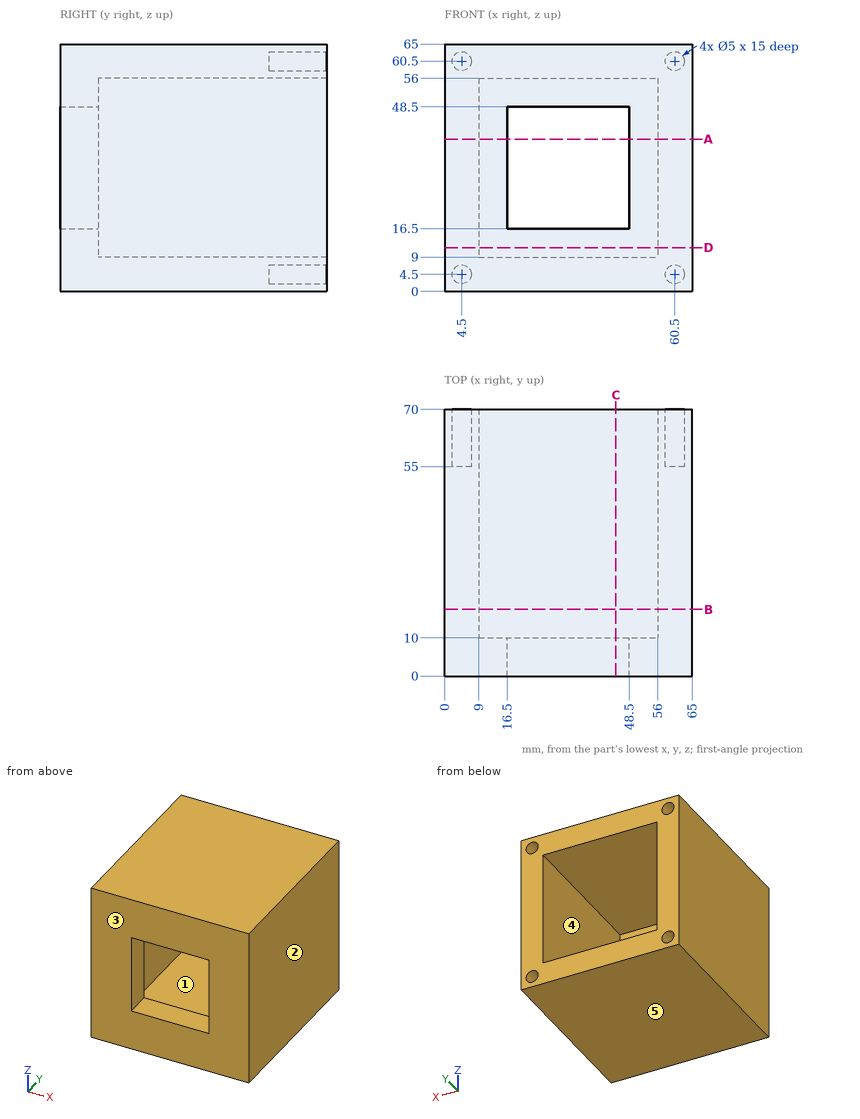
Verification items for this drawing (mm, ordinates from the low corner). A direction names the side the tool comes from. Coordinates: 2 decimals unless noted, no trailing zeros. Order: outer loops, then holes, each group sorted by start corner. A loop starts at its lowest first (then second) coordinate and runs counter-clockwise, first axis right, second up. Notation, with made-up numbers: (63, -13) - (92, -13) arc R16 cw to (92, 1) - close; hole circle Ø11 at (-20.5, 57.5). An arc over 180 degrees is marked (long way). Answer in a Markdown table with one row per item. Add a question column.
1. Gauge pin test, flat ends, axial feed: pin 1 Ø2.5 at (x, z) = (4, 60.5) entering from +Y; pin 2 Ø23.5 at (x, z) = (22, 37) entering from +Y. Record the tip position at first contact, or that the pin passes through.
2. Section check A-A (z = 40). Enter the section's corners in (x, y), plus the area to 3 significant figures.
3. Section check C-C (x = 45). Enter the section's corners in (y, z).
4. Section check D-D (z = 11.5). Enter the section's corners in (x, y).
5. Section check B-B (y = 17.5). Enter the section's corners in (x, z).
6. Draft check along Z on the marked faces 3, 4 and 5. Enter one of: +Z half, -Z half, draft (parallel to the pull), parting line (faces both ways), or undercut.
7. Access from +Z, -Z, +X, -X, +Y, -Y to the whole of each face (thin tool, end or side, straight path). Record for the marked faces 1 and 2.
8. Material ranges on L1, parallel to Z at x = 60.5, y = 65; L2, parallel to X at y = 63.5, z = 18, recorded low to high. Write a range as [from, to].
Data:
| question | item | result |
|---|---|---|
| 1 | pin 1 | stops at y = 55 |
| 1 | pin 2 | stops at y = 10 |
| 2 | outline | (0, 0) - (16.5, 0) - (16.5, 10) - (9, 10) - (9, 70) - (0, 70) - close; (48.5, 0) - (65, 0) - (65, 70) - (56, 70) - (56, 10) - (48.5, 10) - close |
| 2 | area | 1,410 mm² |
| 3 | outline | (0, 0) - (70, 0) - (70, 9) - (10, 9) - (10, 16.5) - (0, 16.5) - close; (0, 48.5) - (10, 48.5) - (10, 56) - (70, 56) - (70, 65) - (0, 65) - close |
| 4 | outline | (0, 0) - (65, 0) - (65, 70) - (56, 70) - (56, 10) - (9, 10) - (9, 70) - (0, 70) - close |
| 5 | outline | (0, 0) - (65, 0) - (65, 65) - (0, 65) - close; hole (9, 9) - (56, 9) - (56, 56) - (9, 56) - close |
| 6 | face 3 | draft |
| 6 | face 4 | undercut |
| 6 | face 5 | -Z half |
| 7 | face 1 | +Y |
| 7 | face 2 | +Z, -Z, +X, +Y, -Y |
| 8 | L1 | z = [0, 2], [7, 58], [63, 65] |
| 8 | L2 | x = [0, 9], [56, 65] |
